Input: part model. Units: mm. Frame: model coordinates. A direction names the side the tool comes from. Round coordinates to 2 decimals unless told otherwise and drop trailing zeros. Order: outer loops, then holes, each group sorted by start corner. A loop starts at its lowest first (then second) coordinate and runs counter-clockwise, first axis right, second up. Notation, with made-up numbers: (-12.75, -8) -> (23.25, -8) arc R14 ccw to (23.25, 10) -> close; hole circle Ø8 at (87, 0.5). An arc over 180 degrees is marked (long way). Answer as CSV lines item,"result". Start each with the question number.
1) Line query: L1, parallel to X at y = -24, z = 1.75; L2, parallel to Y at x = 33.75, z = 1.9; L3, parallel to Y at x = -23.5, z = 1.6. Output: solid intervals per line, ascending.
2) Section query D-D, the plane y = -19.5. Output: boundary loops of the cut face in (x, z), and give its area (3 significant figures).
3) Section query A-A, the plane y = 0.5. Output: boundary loops of the cut face in (x, z).
4) Section query C-C, the plane x = -3. Output: boundary loops of the cut face in (y, z), and give its area (3 significant figures).
5) Section query B-B, the plane y = 10. Output: boundary loops of the cut face in (x, z), and give its area (4 significant figures).
6) Access query for faces 1 (the face through (-10, 25, 2)), 2 (the face through (-38.137, 29.818, 1.726)). Directions: +Z, -Z, +X, -X, +Y, -Y. A direction counts if a zero-diameter tool reaches every point of the face in a straight line with its end or side. Return the directions, or none.
7) First-contact query: P1, Ø1.8, axis at x = -33.5, z = 1, coming from the +Y side; P2, Ø12, axis at x = 17.5, y = 17, coming from the -Z side. Flat tips, straight axial feed; report the tip coordinate or a pass-through.
8) Mould query, pull axis X, two halves, no side actions, for faces 3 (the face through (34, -10, 2)), 4 (the face through (27.25, -25, 2)), 5 (the face through (-5.754, 39.983, 1.726)), 6 (the face through (37.85, -30.14, 1.73)). Classes: +X half, -X half, draft (parallel to the pull), parting line (faces both ways), or undercut.
```python
from build123d import *

# Parameters (mm, degrees)
SKETCH1_R           = 1.5
SKETCH1_W           = 40.5
SKETCH1_H           = 20.5
BOSS_EXTRUDE1_DEPTH = 3.5
SKETCH2_R           = 1.55
SKETCH2_W           = 3.5
SKETCH2_H           = 6
CUT_EXTRUDE1_DEPTH  = 63.568462503
SKETCH3_W           = 15
SKETCH3_H           = 3.5
CUT_EXTRUDE2_DEPTH  = 63.568462503
SKETCH4_R           = 1.5
CUT_EXTRUDE3_DEPTH  = 63.568462503
CUT_EXTRUDE5_REACH  = 64.568
SKETCH5_R           = 1.5
SKETCH6_W           = 30
SKETCH6_H           = 3
CUT_EXTRUDE6_DEPTH  = 10


with BuildPart() as part:
    # Sketch1 → Boss-Extrude1 (new body)
    with BuildSketch(Plane.XY):
        with BuildLine():
            Line((-35.75, -31), (35.75, -31))
            ThreePointArc((35.75, -31), (37.871320344, -30.121320344), (38.75, -28))
            Line((38.75, -28), (38.75, 28))
            ThreePointArc((38.75, 28), (38.657529209, 28.739103444), (38.385817399, 29.432643235))
            Line((38.385817399, 29.432643235), (28.88626309, 46.91019098))
            ThreePointArc((28.88626309, 46.91019098), (26.903491848, 48.695137654), (24.239382807, 48.836344739))
            Line((24.239382807, 48.836344739), (-36.599342813, 30.877258554))
            ThreePointArc((-36.599342813, 30.877258554), (-38.152917855, 29.796102943), (-38.75, 28))
            Line((-38.75, 28), (-38.75, -28))
            ThreePointArc((-38.75, -28), (-37.871320344, -30.121320344), (-35.75, -31))
        make_face()
        with Locations((25.371839891, 45)):
            Circle(SKETCH1_R, mode=Mode.SUBTRACT)
        with Locations((-9.5, 14.75)):
            Rectangle(SKETCH1_W, SKETCH1_H, mode=Mode.SUBTRACT)
    extrude(amount=BOSS_EXTRUDE1_DEPTH)

    # Sketch2 → Cut-Extrude1 (cut, through all)
    with BuildSketch(Plane(origin=(0, 0, 0), x_dir=(-1, 0, 0), z_dir=(0, 0, -1))):
        with Locations((-33.75, -19.5)):
            Circle(SKETCH2_R)
        with Locations(Location((33.75, -19.5, 0), (0, 0, 180))):
            Circle(SKETCH2_R)
        with Locations((-33.75, -13)):
            Rectangle(SKETCH2_W, SKETCH2_H)
        with Locations((-33.75, -26)):
            Rectangle(SKETCH2_W, SKETCH2_H)
        with Locations((33.75, -26)):
            Rectangle(SKETCH2_W, SKETCH2_H)
        with Locations((33.75, -13)):
            Rectangle(SKETCH2_W, SKETCH2_H)
    extrude(amount=-CUT_EXTRUDE1_DEPTH, mode=Mode.SUBTRACT)

    # Sketch3 → Cut-Extrude2 (cut, through all)
    with BuildSketch(Plane(origin=(0, 0, 0), x_dir=(-1, 0, 0), z_dir=(0, 0, -1))):
        with Locations((19.75, -24.75)):
            Rectangle(SKETCH3_W, SKETCH3_H)
        with Locations((-19.75, -24.75)):
            Rectangle(SKETCH3_W, SKETCH3_H)
    extrude(amount=-CUT_EXTRUDE2_DEPTH, mode=Mode.SUBTRACT)

    # Sketch4 → Cut-Extrude3 (cut, through all)
    with BuildSketch(Plane(origin=(0, 0, 0), x_dir=(-1, 0, 0), z_dir=(0, 0, -1))):
        with Locations((-15, 19.5)):
            Circle(SKETCH4_R)
        with Locations((-15, 10)):
            Circle(SKETCH4_R)
        with Locations((34, 10)):
            Circle(SKETCH4_R)
        with Locations((34, 19.5)):
            Circle(SKETCH4_R)
    extrude(amount=-CUT_EXTRUDE3_DEPTH, mode=Mode.SUBTRACT)

    # Sketch5 → Cut-Extrude5 (cut, up to next)
    with BuildSketch(Plane(origin=(0, 0, 0), x_dir=(-1, 0, 0), z_dir=(0, 0, -1)), mode=Mode.PRIVATE) as cut_extrude5_sk1:
        with Locations((34, 0.5)):
            Circle(SKETCH5_R)
    cut_extrude5_tool1 = extrude(cut_extrude5_sk1.sketch, amount=-CUT_EXTRUDE5_REACH, mode=Mode.PRIVATE) & part.part
    add(cut_extrude5_tool1.solids().sort_by_distance((-34, 0.5, 0))[0], mode=Mode.SUBTRACT)

    # Sketch6 → Cut-Extrude6 (cut)
    with BuildSketch(Plane.XY.offset(3.5)):
        with Locations((0, -29.5)):
            Rectangle(SKETCH6_W, SKETCH6_H)
    extrude(amount=-CUT_EXTRUDE6_DEPTH, mode=Mode.SUBTRACT)


solid = part.part
```
Findings:
1,L1,"x = -38.75 to -35.5, -32 to -27.25, -12.25 to 12.25, 27.25 to 32, 35.5 to 38.75"
1,L2,"y = -31 to -29, -23 to -21.05, -17.95 to -16, -10 to 37.96"
1,L3,"y = -31 to -26.5, -23 to 4.5, 25 to 34.74"
2,outline,"(-38.75, 0) -> (-35.3, 0) -> (-35.3, 3.5) -> (-38.75, 3.5) -> close; (-32.2, 0) -> (32.2, 0) -> (32.2, 3.5) -> (-32.2, 3.5) -> close; (35.3, 0) -> (38.75, 0) -> (38.75, 3.5) -> (35.3, 3.5) -> close"
2,area,"250 mm^2"
3,outline,"(-38.75, 0) -> (-35.5, 0) -> (-35.5, 3.5) -> (-38.75, 3.5) -> close; (-32.5, 0) -> (38.75, 0) -> (38.75, 3.5) -> (-32.5, 3.5) -> close"
4,outline,"(-28, 0) -> (4.5, 0) -> (4.5, 3.5) -> (-28, 3.5) -> close; (25, 0) -> (40.8, 0) -> (40.8, 3.5) -> (25, 3.5) -> close"
4,area,"169 mm^2"
5,outline,"(-38.75, 0) -> (-35.5, 0) -> (-35.5, 3.5) -> (-38.75, 3.5) -> close; (-32.5, 0) -> (-29.75, 0) -> (-29.75, 3.5) -> (-32.5, 3.5) -> close; (10.75, 0) -> (13.5, 0) -> (13.5, 3.5) -> (10.75, 3.5) -> close; (16.5, 0) -> (38.75, 0) -> (38.75, 3.5) -> (16.5, 3.5) -> close"
5,area,"108.5 mm^2"
6,face 1,"+Z, -Z"
6,face 2,"+Z, -Z, -X, +Y"
7,P1,"stops at y = 32.06"
7,P2,"stops at z = 0"
8,face 3,"undercut"
8,face 4,"undercut"
8,face 5,"-X half"
8,face 6,"+X half"
